Geometry: final body of the model. Coordinates: model frame, mm. Face numbers are marked on the shaded views. A direction names the side the tool comes from. Give positions to 0.01 mm unless a question says otherwise; leave off trailing zeros. Write each loop counter-clockwise with the first axis right and the second up, starting at its lowest first coordinate (ties: lowest second). Pieces come first, ordered by that corner, then holes.
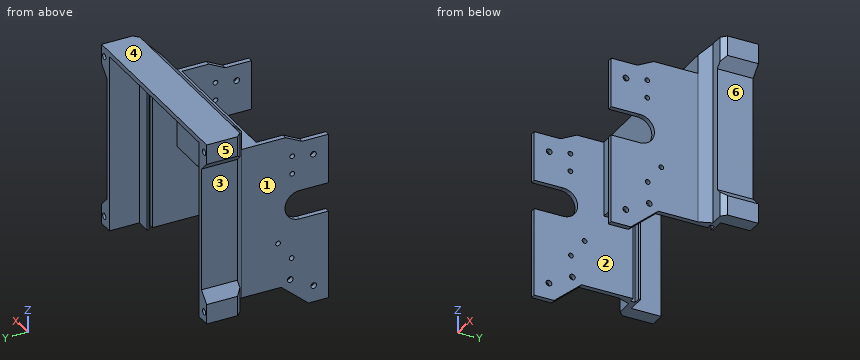
```python
from build123d import *

# Parameters (mm, degrees)
SKETCH_1_W          = 9.5
SKETCH_1_H          = 8
EXTRUDE_1_DEPTH     = 2
SKETCH_2_R          = 1.15
SKETCH_2_R_2        = 0.95
CUT_EXTRUDE_1_DEPTH = 40.502623296
SKETCH_3_W          = 2
SKETCH_3_H          = 61.22
EXTRUDE_2_DEPTH     = 6
SKETCH_4_W          = 61.22
SKETCH_4_H          = 2
EXTRUDE_3_DEPTH     = 58.3
EXTRUDE_START       = -2
SKETCH_5_R          = 0.95
SKETCH_5_R_2        = 1.15
EXTRUDE_4_DEPTH     = 2
EXTRUDE_5_DEPTH     = 61.22
EXTRUDE_6_DEPTH     = 2
SKETCH_10_W         = 1.85
SKETCH_10_H         = 59.22
CUT_EXTRUDE_2_DEPTH = 0.2
SKETCH_11_W         = 0.12
SKETCH_11_H         = 1.8
CUT_EXTRUDE_4_DEPTH = 59.22
CUT_EXTRUDE_START   = -30.82
SKETCH_12_W         = 56.3
SKETCH_12_H         = 2
CUT_EXTRUDE_5_DEPTH = 30.82
EXTRUDE_7_DEPTH     = 10.6
SKETCH_14_W         = 71.82
SKETCH_14_H         = 2.4
EXTRUDE_8_DEPTH     = 1.32
SKETCH_15_W         = 71.82
SKETCH_15_H         = 2.4
EXTRUDE_9_DEPTH     = 2.48
EXTRUDE_10_DEPTH    = 2
SKETCH_17_W         = 73.82
SKETCH_17_H         = 2.4
EXTRUDE_11_DEPTH    = 2
SKETCH_18_W         = 73.82
SKETCH_18_H         = 2.4
EXTRUDE_12_DEPTH    = 2
EXTRUDE_13_DEPTH    = 12
SKETCH_20_W         = 4
SKETCH_20_H         = 8
SKETCH_20_R         = 1.2
EXTRUDE_14_DEPTH    = 10
SKETCH_21_W         = 4
SKETCH_21_H         = 8
EXTRUDE_15_DEPTH    = 3
SKETCH_22_W         = 4
SKETCH_22_H         = 8
EXTRUDE_16_DEPTH    = 4.4
CHAMFER_1_SIZE      = 4
CHAMFER_2_SIZE      = 2
CHAMFER_3_SIZE      = 5


with BuildPart() as part:
    # 草图1 → 凸台-拉伸1 (new body)
    with BuildSketch(Plane(origin=(0, 0, 0), x_dir=(0, 0, -1), z_dir=(1, 0, 0))):
        with BuildLine():
            Line((-2, -13.637332849), (24.2, -13.637332849))
            Line((24.2, -13.637332849), (24.2, -5.637332849))
            Line((24.2, -5.637332849), (24.2, 5.362667151))
            Line((24.2, 5.362667151), (24.2, 10.362667151))
            Line((24.2, 10.362667151), (-37.02, 10.362667151))
            Line((-37.02, 10.362667151), (-37.02, 3.562667151))
            Line((-37.02, 3.562667151), (-33.7, -3.037332849))
            Line((-33.7, -3.037332849), (-33.7, -13.637332849))
            Line((-33.7, -13.637332849), (-13.7, -13.637332849))
            Line((-13.7, -13.637332849), (-13.7, -2.037332849))
            ThreePointArc((-13.7, -2.037332849), (-7.85, 3.812667151), (-2, -2.037332849))
            Line((-2, -2.037332849), (-2, -13.637332849))
        make_face()
        Polygon((24.2, -5.637332849), (33.7, -5.637332849), (24.2, 5.362667151), align=None)
        with Locations((28.95, -9.637332849)):
            Rectangle(SKETCH_1_W, SKETCH_1_H)
    extrude(amount=EXTRUDE_1_DEPTH)

    # 草图2 → 切除-拉伸1 (cut, through all)
    with BuildSketch(Plane(origin=(2, 0, 0), x_dir=(0, 0, -1), z_dir=(1, 0, 0))):
        with Locations((27.12, -7.727332849)):
            Circle(SKETCH_2_R)
        with Locations((-27.12, -7.627332849)):
            Circle(SKETCH_2_R)
        with Locations((22, 1.712667151)):
            Circle(SKETCH_2_R)
        with Locations((13.31, 1.112667151)):
            Circle(SKETCH_2_R_2)
        with Locations((5.79, 6.592667151)):
            Circle(SKETCH_2_R_2)
        with Locations((-21.41, 0.912667151)):
            Circle(SKETCH_2_R_2)
        with Locations((-28.63, 0.912667151)):
            Circle(SKETCH_2_R_2)
    extrude(amount=-CUT_EXTRUDE_1_DEPTH, mode=Mode.SUBTRACT)

    # 草图3 → 凸台-拉伸2 (add)
    with BuildSketch(Plane(origin=(0, 10.362667151, 0), x_dir=(1, 0, 0), z_dir=(0, 1, 0))):
        with Locations((1, -6.41)):
            Rectangle(SKETCH_3_W, SKETCH_3_H)
    extrude(amount=EXTRUDE_2_DEPTH)

    # 草图4 → 凸台-拉伸3 (add)
    with BuildSketch(Plane.ZY):
        with Locations((6.41, 15.362667151)):
            Rectangle(SKETCH_4_W, SKETCH_4_H)
    extrude(amount=EXTRUDE_3_DEPTH)

    # 草图5 → 凸台-拉伸4 (add)
    with BuildSketch(Plane.ZY.offset(58.3).offset(EXTRUDE_START)):
        with BuildLine():
            Line((37.02, 14.362667151), (-24.2, 14.362667151))
            Line((-24.2, 14.362667151), (-24.2, 5.362667151))
            Line((-24.2, 5.362667151), (-33.7, -5.637332849))
            Line((-33.7, -5.637332849), (-33.7, -13.637332849))
            Line((-33.7, -13.637332849), (2, -13.637332849))
            Line((2, -13.637332849), (2, -2.037332849))
            ThreePointArc((2, -2.037332849), (7.85, 3.812667151), (13.7, -2.037332849))
            Line((13.7, -2.037332849), (13.7, -13.637332849))
            Line((13.7, -13.637332849), (33.7, -13.637332849))
            Line((33.7, -13.637332849), (33.7, -3.037332849))
            Line((33.7, -3.037332849), (37.02, 3.562667151))
            Line((37.02, 3.562667151), (37.02, 14.362667151))
        make_face()
        with Locations(Location((-13.31, 1.112667151, 0), (0, 0, 180))):
            Circle(SKETCH_5_R, mode=Mode.SUBTRACT)
        with Locations(Location((-22, 1.712667151, 0), (0, 0, 180))):
            Circle(SKETCH_5_R_2, mode=Mode.SUBTRACT)
        with Locations(Location((-27.12, -7.727332849, 0), (0, 0, 180))):
            Circle(SKETCH_5_R_2, mode=Mode.SUBTRACT)
        with Locations(Location((-5.79, 6.592667151, 0), (0, 0, 180))):
            Circle(SKETCH_5_R, mode=Mode.SUBTRACT)
        with Locations(Location((21.41, 0.912667151, 0), (0, 0, 180))):
            Circle(SKETCH_5_R, mode=Mode.SUBTRACT)
        with Locations(Location((28.63, 0.912667151, 0), (0, 0, 180))):
            Circle(SKETCH_5_R, mode=Mode.SUBTRACT)
        with Locations(Location((27.12, -7.627332849, 0), (0, 0, 180))):
            Circle(SKETCH_5_R_2, mode=Mode.SUBTRACT)
    extrude(amount=EXTRUDE_4_DEPTH)

    # 草图7 → 凸台-拉伸5 (add)
    with BuildSketch(Plane.XY.offset(37.02)):
        Polygon((-58.3, 21.362667151), (-58.3, 16.362667151), (-56.3, 16.362667151), (-56.3, 26.362667151), (-58.15, 26.362667151), (-58.15, 27.962667151), (-55.65, 27.962667151), (-55.65, 28.762667151), (-60.15, 28.762667151), (-60.15, 26.362667151), align=None)
        Polygon((0, 26.362667151), (0, 16.362667151), (2, 16.362667151), (2, 21.362667151), (3.85, 26.362667151), (3.85, 28.762667151), (-0.65, 28.762667151), (-0.65, 27.962667151), (1.85, 27.962667151), (1.85, 26.362667151), align=None)
    extrude(amount=-EXTRUDE_5_DEPTH)

    # 草图8 → 凸台-拉伸6 (add)
    with BuildSketch(Plane.XY.offset(37.02)):
        Polygon((-55.65, 28.762667151), (-0.65, 28.762667151), (-0.65, 27.962667151), (1.85, 27.962667151), (1.85, 26.362667151), (0, 26.362667151), (0, 16.362667151), (-56.3, 16.362667151), (-56.3, 26.362667151), (-58.15, 26.362667151), (-58.15, 27.962667151), (-55.65, 27.962667151), align=None)
        Polygon((0, 26.362667151), (0, 16.362667151), (-56.3, 16.362667151), (-56.3, 26.362667151), (-58.15, 26.362667151), (-58.15, 27.962667151), (-55.65, 27.962667151), (-55.65, 28.762667151), (-60.15, 28.762667151), (-60.15, 26.362667151), (-58.3, 21.362667151), (-58.3, 3.562667151), (-56.3, 3.562667151), (-56.3, 14.362667151), (0, 14.362667151), (0, 3.562667151), (2, 3.562667151), (2, 21.362667151), (3.85, 26.362667151), (3.85, 28.762667151), (-0.65, 28.762667151), (-0.65, 27.962667151), (1.85, 27.962667151), (1.85, 26.362667151), align=None)
    extrude(amount=-EXTRUDE_6_DEPTH)

    # 草图10 → 切除-拉伸2 (cut)
    with BuildSketch(Plane(origin=(0, 26.362667151, 0), x_dir=(1, 0, 0), z_dir=(0, 1, 0))):
        with Locations((0.925, -5.41)):
            Rectangle(SKETCH_10_W, SKETCH_10_H)
        with Locations((-57.225, -5.41)):
            Rectangle(SKETCH_10_W, SKETCH_10_H)
    extrude(amount=-CUT_EXTRUDE_2_DEPTH, mode=Mode.SUBTRACT)

    # 草图11 → 切除-拉伸4 (cut)
    with BuildSketch(Plane(origin=(0, 0, -24.2), x_dir=(-1, 0, 0), z_dir=(0, 0, -1))):
        with Locations((-1.91, 27.062667151)):
            Rectangle(SKETCH_11_W, SKETCH_11_H)
        with Locations((58.21, 27.062667151)):
            Rectangle(SKETCH_11_W, SKETCH_11_H)
    extrude(amount=-CUT_EXTRUDE_4_DEPTH, mode=Mode.SUBTRACT)

    # 草图12 → 切除-拉伸5 (cut)
    with BuildSketch(Plane(origin=(0, 0, -24.2), x_dir=(-1, 0, 0), z_dir=(0, 0, -1)).offset(CUT_EXTRUDE_START)):
        with Locations((28.15, 15.362667151)):
            Rectangle(SKETCH_12_W, SKETCH_12_H)
    extrude(amount=CUT_EXTRUDE_5_DEPTH, mode=Mode.SUBTRACT)

    # 草图13 → 凸台-拉伸7 (add)
    with BuildSketch(Plane.XY.offset(37.02)):
        Polygon((-58.3, 21.362667151), (2, 21.362667151), (3.85, 26.362667151), (3.85, 28.762667151), (-60.15, 28.762667151), (-60.15, 26.362667151), align=None)
    extrude(amount=EXTRUDE_7_DEPTH)

    # 草图14 → 凸台-拉伸8 (add)
    with BuildSketch(Plane(origin=(3.85, 0, 0), x_dir=(0, 0, -1), z_dir=(1, 0, 0))):
        with Locations((-11.71, 27.562667151)):
            Rectangle(SKETCH_14_W, SKETCH_14_H)
    extrude(amount=EXTRUDE_8_DEPTH)

    # 草图15 → 凸台-拉伸9 (add)
    with BuildSketch(Plane.ZY.offset(60.15)):
        with Locations((11.71, 27.562667151)):
            Rectangle(SKETCH_15_W, SKETCH_15_H)
    extrude(amount=EXTRUDE_9_DEPTH)

    # 草图16 → 凸台-拉伸10 (add)
    with BuildSketch(Plane.XY.offset(47.62)):
        Polygon((-58.3, 21.362667151), (2, 21.362667151), (3.85, 26.362667151), (5.17, 26.362667151), (5.17, 28.762667151), (-62.63, 28.762667151), (-62.63, 26.362667151), (-60.15, 26.362667151), align=None)
    extrude(amount=EXTRUDE_10_DEPTH)

    # 草图17 → 凸台-拉伸11 (add)
    with BuildSketch(Plane(origin=(5.17, 0, 0), x_dir=(0, 0, -1), z_dir=(1, 0, 0))):
        with Locations((-12.71, 27.562667151)):
            Rectangle(SKETCH_17_W, SKETCH_17_H)
    extrude(amount=EXTRUDE_11_DEPTH)

    # 草图18 → 凸台-拉伸12 (add)
    with BuildSketch(Plane.ZY.offset(62.63)):
        with Locations((12.71, 27.562667151)):
            Rectangle(SKETCH_18_W, SKETCH_18_H)
    extrude(amount=EXTRUDE_12_DEPTH)

    # 草图19 → 凸台-拉伸13 (add)
    with BuildSketch(Plane(origin=(0, 28.762667151, 0), x_dir=(1, 0, 0), z_dir=(0, 1, 0))):
        Polygon((-62.63, -47.62), (-62.63, 22.2), (-62.63, 24.2), (-64.63, 24.2), (-64.63, -49.62), (7.17, -49.62), (7.17, 24.2), (5.17, 24.2), (5.17, 22.2), (5.17, -47.62), align=None)
    extrude(amount=EXTRUDE_13_DEPTH)

    # 草图20 → 凸台-拉伸14 (add)
    # profile 1 of 4: a face of its own
    with BuildSketch(Plane(origin=(0, 40.762667151, 0), x_dir=(1, 0, 0), z_dir=(0, 1, 0))):
        with Locations((-66.63, -45.62)):
            Rectangle(SKETCH_20_W, SKETCH_20_H)
        with Locations(Location((-66.63, -45.62, 0), (0, 0, 270))):
            Circle(SKETCH_20_R, mode=Mode.SUBTRACT)
    # profile 2 of 4: a face of its own
    with BuildSketch(Plane(origin=(0, 40.762667151, 0), x_dir=(1, 0, 0), z_dir=(0, 1, 0))):
        with Locations((9.17, -45.62)):
            Rectangle(SKETCH_20_W, SKETCH_20_H)
        with Locations(Location((9.17, -45.62, 0), (0, 0, 270))):
            Circle(SKETCH_20_R, mode=Mode.SUBTRACT)
    # profile 3 of 4: a face of its own
    with BuildSketch(Plane(origin=(0, 40.762667151, 0), x_dir=(1, 0, 0), z_dir=(0, 1, 0))):
        with Locations((-66.63, 20.2)):
            Rectangle(SKETCH_20_W, SKETCH_20_H)
        with Locations(Location((-66.63, 20.2, 0), (0, 0, 270))):
            Circle(SKETCH_20_R, mode=Mode.SUBTRACT)
    # profile 4 of 4: a face of its own
    with BuildSketch(Plane(origin=(0, 40.762667151, 0), x_dir=(1, 0, 0), z_dir=(0, 1, 0))):
        with Locations((9.17, 20.2)):
            Rectangle(SKETCH_20_W, SKETCH_20_H)
        with Locations(Location((9.17, 20.2, 0), (0, 0, 270))):
            Circle(SKETCH_20_R, mode=Mode.SUBTRACT)
    extrude(amount=-EXTRUDE_14_DEPTH)

    # 草图21 → 凸台-拉伸15 (add)
    with BuildSketch(Plane.XZ.offset(-30.762667151)):
        with Locations((-66.63, -20.2)):
            Rectangle(SKETCH_21_W, SKETCH_21_H)
        with Locations((-66.63, 45.62)):
            Rectangle(SKETCH_21_W, SKETCH_21_H)
        with Locations((9.17, -20.2)):
            Rectangle(SKETCH_21_W, SKETCH_21_H)
        with Locations((9.17, 45.62)):
            Rectangle(SKETCH_21_W, SKETCH_21_H)
    extrude(amount=-EXTRUDE_15_DEPTH)

    # 草图22 → 凸台-拉伸16 (add)
    with BuildSketch(Plane.XZ.offset(-30.762667151)):
        with Locations((-66.63, 45.62)):
            Rectangle(SKETCH_22_W, SKETCH_22_H)
        with Locations((-66.63, -20.2)):
            Rectangle(SKETCH_22_W, SKETCH_22_H)
        with Locations((9.17, -20.2)):
            Rectangle(SKETCH_22_W, SKETCH_22_H)
        with Locations((9.17, 45.62)):
            Rectangle(SKETCH_22_W, SKETCH_22_H)
    extrude(amount=EXTRUDE_16_DEPTH)

    # 倒角1
    chamfer_1_edges = [part.edges().sort_by_distance(p)[0] for p in [
        (-64.63, 33.562667151, 41.62),
        (7.17, 33.562667151, 41.62),
        (-64.63, 33.562667151, -16.2),
        (7.17, 33.562667151, -16.2),
    ]]
    chamfer(chamfer_1_edges, length=CHAMFER_1_SIZE - 0.0001)  # a hair under: the kernel refuses the full size

    # 倒角2
    chamfer_2_edges = [part.edges().sort_by_distance(p)[0] for p in [
        (-68.63, 26.362667151, 45.62),
        (-68.63, 26.362667151, -20.2),
        (11.17, 26.362667151, -20.2),
        (11.17, 26.362667151, 45.62),
    ]]
    chamfer(chamfer_2_edges, length=CHAMFER_2_SIZE)

    # 倒角3
    chamfer_3_edges = [part.edges().sort_by_distance(p)[0] for p in [
        (-28.15, 21.362667151, 49.62),
    ]]
    chamfer(chamfer_3_edges, length=CHAMFER_3_SIZE)


solid = part.part
```
Item 1: Reachability of the marked faces 1, 2 and 3 from +Z, -Z, +X, -X, +Y, -Y: full face, straight path, thin tool, end or side. Return the list, or none.
Found:
face 1: +Z, -Z, -X, -Y
face 2: -Z
face 3: -X, +Y, -Y
Item 2: Pin query (flat end, axial travel): pin 1 Ø2 at (y, z) = (-7.73, -27.12) entering from -X; pin 2 Ø10 at (x, z) = (-27, 25) entering from +Y; pin 3 Ø10 at (x, y) = (2, 6) entering from -Z; pin 4 Ø6 at (x, y) = (-29.5, 25.5) entering from -Z. Return the tip coordinate at first contact, or that it passes through.
Found:
pin 1: passes through
pin 2: stops at y = 16.36
pin 3: stops at z = -27.97
pin 4: stops at z = 35.02
Item 3: Section B-B, the plane z = -11. Return the cut outline in (x, y).
Found:
outline: (-64.63, 26.36) - (-60.15, 26.36) - (-58.3, 21.36) - (-58.3, -13.64) - (-56.3, -13.64) - (-56.3, 26.16) - (-58.27, 26.16) - (-58.27, 27.96) - (-55.65, 27.96) - (-55.65, 28.76) - (-62.63, 28.76) - (-62.63, 40.76) - (-64.63, 40.76) - close; (-0.65, 27.96) - (1.97, 27.96) - (1.97, 26.16) - (0, 26.16) - (0, -13.64) - (2, -13.64) - (2, 21.36) - (3.85, 26.36) - (7.17, 26.36) - (7.17, 40.76) - (5.17, 40.76) - (5.17, 28.76) - (-0.65, 28.76) - close
Item 4: Section C-C, the plane y = 12. Return the cut outline in (x, z), plus the area to 3 significant figures.
Found:
outline: (-58.3, -24.2) - (-56.3, -24.2) - (-56.3, 37.02) - (-58.3, 37.02) - close; (0, -24.2) - (2, -24.2) - (2, 37.02) - (0, 37.02) - close
area: 245 mm2
Item 5: Section A-A, the plane y = -10. Return the cut outline in (x, z), plus the area to 3 significant figures.
Found:
outline: (-58.3, -33.7) - (-56.3, -33.7) - (-56.3, 2) - (-58.3, 2) - close; (-58.3, 13.7) - (-56.3, 13.7) - (-56.3, 33.7) - (-58.3, 33.7) - close; (0, -33.7) - (2, -33.7) - (2, 2) - (0, 2) - close; (0, 13.7) - (2, 13.7) - (2, 33.7) - (0, 33.7) - close
area: 223 mm2
Item 6: Line query: L1, parallel to Y at x = -56.9, z = 28.63; L2, parallel to X at y = 38, z = 45.62; L3, parallel to Y at x = 1.6, z = -22. Output: solid intervals per line, ascending.
Found:
L1: y = -13.64 to -0.04, 1.86 to 26.16, 27.96 to 28.76
L2: x = -68.63 to -67.83, -65.43 to -62.63, 5.17 to 7.97, 10.37 to 11.17
L3: y = -13.64 to 0.56, 2.86 to 26.16, 27.96 to 28.76
Item 7: Pull-direction query (Z, two-part tool) for the marked faces 4, 5 and 6; classes: +Z half, -Z half, draft (parallel to the pull), parting line (faces both ways), or undercut.
Found:
face 4: +Z half
face 5: draft
face 6: undercut
